```python
from build123d import *

# Parameters (mm, degrees)
REVOLVE1_ANGLE     = 270
SKETCH11_R         = 7.5
CUT_EXTRUDE1_DEPTH = 103


with BuildPart() as part:
    # Sketch10 → Revolve1 (revolve)
    with BuildSketch(Plane.XY):
        with BuildLine():
            Line((-146.868713488, 1.727510523), (-96.868713488, 1.727510523))
            Line((-96.868713488, 1.727510523), (-96.868713488, 12.246455007))
            Line((-96.868713488, 12.246455007), (3.131286512, 12.246455007))
            Line((3.131286512, 12.246455007), (3.131286512, 27.246455007))
            Line((3.131286512, 27.246455007), (-16.868713488, 27.246455007))
            Line((-16.868713488, 27.246455007), (-16.868713488, 48.546455007))
            Line((-16.868713488, 48.546455007), (-26.868713488, 48.546455007))
            Line((-26.868713488, 48.546455007), (-26.868713488, 30.664510563))
            Line((-26.868713488, 30.664510563), (-31.868713488, 30.664510563))
            Line((-31.868713488, 30.664510563), (-31.868713488, 55.369461788))
            ThreePointArc((-31.868713488, 55.369461788), (-33.10183862, 56.333258752), (-34.368713488, 57.252242021))
            Line((-34.368713488, 57.252242021), (-34.368713488, 30.664510563))
            Line((-34.368713488, 30.664510563), (-39.368713488, 30.664510563))
            Line((-39.368713488, 30.664510563), (-39.368713488, 60.267954644))
            ThreePointArc((-39.368713488, 60.267954644), (-40.609283081, 60.882526075), (-41.868713488, 61.457457384))
            Line((-41.868713488, 61.457457384), (-41.868713488, 30.664510563))
            Line((-41.868713488, 30.664510563), (-46.868713488, 30.664510563))
            Line((-46.868713488, 30.664510563), (-46.868713488, 63.290372193))
            ThreePointArc((-46.868713488, 63.290372193), (-48.113771821, 63.642379564), (-49.368713488, 63.957341236))
            Line((-49.368713488, 63.957341236), (-49.368713488, 30.664510563))
            Line((-49.368713488, 30.664510563), (-54.368713488, 30.664510563))
            Line((-54.368713488, 30.664510563), (-54.368713488, 64.830682747))
            ThreePointArc((-54.368713488, 64.830682747), (-55.617164341, 64.956446576), (-56.868713488, 65.046284243))
            Line((-56.868713488, 65.046284243), (-56.868713488, 30.664510563))
            Line((-56.868713488, 30.664510563), (-61.868713488, 30.664510563))
            Line((-61.868713488, 30.664510563), (-61.868713488, 65.046284243))
            ThreePointArc((-61.868713488, 65.046284243), (-63.120262635, 64.956446576), (-64.368713488, 64.830682747))
            Line((-64.368713488, 64.830682747), (-64.368713488, 30.664510563))
            Line((-64.368713488, 30.664510563), (-69.368713488, 30.664510563))
            Line((-69.368713488, 30.664510563), (-69.368713488, 63.957341236))
            ThreePointArc((-69.368713488, 63.957341236), (-70.623655155, 63.642379564), (-71.868713488, 63.290372193))
            Line((-71.868713488, 63.290372193), (-71.868713488, 30.664510563))
            Line((-71.868713488, 30.664510563), (-76.868713488, 30.664510563))
            Line((-76.868713488, 30.664510563), (-76.868713488, 61.457457384))
            ThreePointArc((-76.868713488, 61.457457384), (-78.128143895, 60.882526075), (-79.368713488, 60.267954644))
            Line((-79.368713488, 60.267954644), (-79.368713488, 30.664510563))
            Line((-79.368713488, 30.664510563), (-84.368713488, 30.664510563))
            Line((-84.368713488, 30.664510563), (-84.368713488, 57.252242021))
            ThreePointArc((-84.368713488, 57.252242021), (-85.635588357, 56.333258752), (-86.868713488, 55.369461788))
            Line((-86.868713488, 55.369461788), (-86.868713488, 30.664510563))
            Line((-86.868713488, 30.664510563), (-91.868713488, 30.664510563))
            Line((-91.868713488, 30.664510563), (-91.868713488, 48.546455007))
            Line((-91.868713488, 48.546455007), (-106.868713488, 48.546455007))
            Line((-106.868713488, 48.546455007), (-121.791389794, 38.480982745))
            Line((-121.791389794, 38.480982745), (-121.791389794, 21.727510523))
            ThreePointArc((-121.791389794, 21.727510523), (-124.720321982, 14.656442711), (-131.791389794, 11.727510523))
            Line((-131.791389794, 11.727510523), (-136.868713488, 11.727510523))
            Line((-136.868713488, 11.727510523), (-136.868713488, 21.727510523))
            Line((-136.868713488, 21.727510523), (-146.868713488, 21.727510523))
            Line((-146.868713488, 21.727510523), (-146.868713488, 1.727510523))
        make_face()
    revolve(axis=Axis((-146.868713488, -13.272489477, 0), (1, 0, 0)), revolution_arc=REVOLVE1_ANGLE)

    # Sketch11 → Cut-Extrude1 (cut)
    with BuildSketch(Plane(origin=(0, 0, 0), x_dir=(-1, 0, 0), z_dir=(0, 0, -1))):
        with Locations((59.368713488, -0.513017235)):
            Circle(SKETCH11_R)
    extrude(amount=-CUT_EXTRUDE1_DEPTH, mode=Mode.SUBTRACT)


solid = part.part
```
Check sheet for the modelled part. Datum: model origin and axes. Units: mm. A direction names the side the tool comes from. Give positions to 0.01 mm unless a question says otherwise; leave off trailing zeros. Loops run counter-clockwise (first coordinate to the right, second up) from the corner with the lowest first, then second, coordinate; pieces in that order, holes last. Notation, with made-up numbers: (67.5, 32.5) - (125.5, 32.5) arc R15 ccw to (125.5, 39.5) - close; hole circle Ø11 at (-0.5, -17). An arc over 180 degrees is marked (long way). One line per question, with ' | ' between items. Start each with the question number.
1. Cross-section at D-D, the plane x = -118.5. Enter the section's corners in (y, z).
2. Draft check along X on faces 1 (the flat face through (-96.869, -24, 12)), 2 (the cylindrical face through (-21.94, -55.52, 45.13)), 3 (the cylindrical face through (-29.404, -43.299, 32.076)). Enter one of: released by +X, released by -X, zero draft, split by the parting line, or undercut.
3. Cross-section at A-A, the plane y = -69. Give the number of separate pieces and of enclosed holes in the cut face, plus the area to 3 significant figures.
4. Set-up check for faces 4 (the flat face through (-64.369, -59, 1)), 5 (the flat face through (-73, -13.272, -40)), 6 (the cylindrical face through (-141.939, -37.192, 25.552)), 7 (the flat face through (-61.869, 36, 38)), 8 (the flat face through (-71.869, -48, 35)): record each of +Z, -Z, +X, -X, +Y, -Y from which the full face is reachable in a straight line by a thin tool's end or side.
5. Material ranges on line 1 along X through (y, z) = (-45, -64.5); line 2 along X through (y, z) = (-26.5, 37); line 3 along X through (y, z) = (-77, -38), recorded low to high. Write a range as [from, to].
6. Gauge pin test, flat ends, axial feed: pin 1 Ø12 at (x, y) = (-28.5, -32.5) entering from -Z; pin 2 Ø6 at (x, y) = (-45.5, -10.5) entering from +Z; pin 3 Ø19 at (x, z) = (-46.5, -54.5) entering from +Y. Record the tip position at first contact, or that the pin passes through.
Check result:
1) outline: (-13.27, -53.97) - (-13.27, -15) arc R15 cw (long way) to (1.73, 0) - (40.7, 0) arc R53.97 ccw (long way) to start
2) face 1: released by +X | face 2: zero draft | face 3: undercut
3) separate pieces: 10 | enclosed holes: 0 | area: 3,640 mm2
4) face 4: -Y | face 5: -Z, +X, -X, +Y | face 6: -X | face 7: +Z, +Y | face 8: none
5) line 1: x = [-79.37, -76.87], [-71.87, -69.37], [-64.37, -61.87], [-56.87, -54.37], [-49.37, -46.87], [-41.87, -39.37] | line 2: x = [-121.79, 3.13] | line 3: x = [-78.04, -76.87], [-71.87, -69.37], [-64.37, -61.87], [-56.87, -54.37], [-49.37, -46.87], [-41.87, -40.7]
6) pin 1: stops at z = -68.23 | pin 2: stops at z = 76.97 | pin 3: stops at y = -13.27
